Input: part model. Units: mm. Frame: model coordinates. A direction names the side the tool comes from. Round coordinates to 2 decimals unless told otherwise and drop trailing zeros. Loops run counter-clockwise (first coordinate to the right, second up) from the corner with the lowest first, then second, coordinate; pieces in that order, holes last. Notation, with made-up numbers: (-8, 41.5) -> (-2, 41.5) arc R27 cw to (-2, 63.5) -> close; hole circle Ø11 at (28, 45.5). An arc over 180 degrees is marked (long way). Answer in a Markdown table with one row per item. Add a question column.
Q1. Section B-B, the plane x = -37. Give the number of separate pieces and of enclosed holes in the cut face, and give its area (3 significant figures).
Q2. Reachability of faces 5 (the face through (-35, 1.5, -14)), 6 (the face through (-29.584, -2.107, 24.79)), 7 (the face through (-35, -6, 0)) from +Z, -Z, +X, -X, +Y, -Y: full face, straight path, thin tool, end or side. Return the list, or none.
Q3. Section D-D, the plane x = -28.25. Output: boundary loops of the cut face in (y, z), and give its area (3 significant figures).
Q4. Mould query, pull axis Z, two halves, no side actions, for faces 1 (the face through (-35, -1.494, -14)), 2 (the face through (-34.59, -0.03, -6.16)), 3 (the face through (-35, -6, 10)), 4 (the face through (-29.584, 2.107, -14.79)). Classes: pulls with the +Z half, pulls with the -Z half, needs draft (parallel to the pull), parting line crosses it, or undercut.
Q5. Pin query (flat end, axial travel): pin 1 (8 mm diameter, centred on x = -31.5, z = 28, fed in from +Y); pin 2 (5 mm diameter, centred on y = 2.5, z = -17, fed in from -X); pin 3 (8.5 mm diameter, centred on x = -37, z = -16.5, fed in from -Y). Return the tip coordinate at first contact, or that it passes through.
Q6. Section A-A, the plane z = 21.5. Output: boundary loops of the cut face in (x, y).
Q7. Ray query, L1, parallel to Z at x = -32, y = -0.25; L2, parallel to X at y = 0, z = 15.5; L3, parallel to Y at x = -34.75, z = -22. Return the intervals inside material, ascending. Write a range as from..to.
Q8. Section C-C, the plane z = -1.5. Output: boundary loops of the cut face in (x, y), and give its area (3 significant figures).
```python
from build123d import *

# Parameters (mm, degrees)
F0_R          = 8.5
F1_DEPTH      = 10
F2_R          = 5.5
F3_DEPTH      = 32
F4_R          = 5.5
F5_DEPTH      = 32
F6_SIZE       = 2
F7_SIZE       = 2
F8_R          = 3.0547772324
F9_DEPTH      = 8.501
F9_DEPTH_BACK = 8.501
F11_DEPTH     = 43.1654968794
F13_DEPTH     = 43.1654968794


with BuildPart() as f1:
    # F0 (on Top) → F1 (new body)
    with BuildSketch(Plane.XY):
        with Locations((-34.6644967794, 0)):
            Circle(F0_R)
    extrude(amount=F1_DEPTH)

    # F2 (on face) → F3 (join)
    with BuildSketch(Plane.XY.offset(10)):
        with Locations((-34.6644967794, 0)):
            Circle(F2_R)
    extrude(amount=F3_DEPTH)

    # F4 (on face) → F5 (join)
    with BuildSketch(Plane(origin=(0, 0, 0), x_dir=(1, 0, 0), z_dir=(0, 0, -1))):
        with Locations((-34.6644967794, 0)):
            Circle(F4_R)
    extrude(amount=F5_DEPTH)

    # F6
    f6_edges = [f1.edges().sort_by_distance(p)[0] for p in [
        (-40.164497, 0, 42),
    ]]
    chamfer(f6_edges, length=F6_SIZE)

    # F7
    f7_edges = [f1.edges().sort_by_distance(p)[0] for p in [
        (-40.164497, 0, -32),
    ]]
    chamfer(f7_edges, length=F7_SIZE)

    # F8 (on Front) → F9 (cut, two sides)
    with BuildSketch(Plane.XZ) as f9_sk:
        with Locations((-34.5804058015, 5.2290405147)):
            Circle(F8_R)
    extrude(amount=-F9_DEPTH, mode=Mode.SUBTRACT)
    extrude(f9_sk.sketch, amount=F9_DEPTH_BACK, mode=Mode.SUBTRACT)

    # F10 (on Right) → F11 (cut, through all)
    with BuildSketch(Plane.YZ):
        with BuildLine():
            Line((1.5, 20.7730699331), (1.5, 32.7730699331))
            ThreePointArc((1.5, 32.7730699331), (-0.0205803002, 34.2729287435), (-1.4994352683, 32.731913207))
            Line((-1.4994352683, 32.731913207), (-1.4994352683, 20.8142266592))
            Line((-1.4994352683, 20.8142266592), (-1.4994352683, 20.731913207))
            ThreePointArc((-1.4994352683, 20.731913207), (0.0205803002, 19.2732111226), (1.5, 20.7730699331))
        make_face()
        with BuildLine():
            Line((-1.4994352683, 20.731913207), (-1.4994352683, 20.8142266592))
            ThreePointArc((-1.4994352683, 20.8142266592), (-1.5, 20.7730699331), (-1.4994352683, 20.731913207))
        make_face()
    extrude(amount=-F11_DEPTH, mode=Mode.SUBTRACT)

    # F12 (on Right) → F13 (cut, through all)
    with BuildSketch(Plane.YZ):
        with BuildLine():
            Line((-1.4940902409, -19.792623133), (-1.4940902409, -19.5265828961))
            ThreePointArc((-1.4940902409, -19.5265828961), (-1.5, -19.6596030146), (-1.4940902409, -19.792623133))
        make_face()
        with BuildLine():
            Line((-1.4940902409, -7.792623133), (-1.4940902409, -19.5265828961))
            Line((-1.4940902409, -19.5265828961), (-1.4940902409, -19.792623133))
            ThreePointArc((-1.4940902409, -19.792623133), (0.0669880568, -21.1581064681), (1.4999997728, -19.6587774142))
            Line((1.4999997728, -19.6587774142), (1.5, -7.6596030146))
            ThreePointArc((1.5, -7.659603043), (-0.0665756517, -6.161081182), (-1.4940902409, -7.792623133))
        make_face()
    extrude(amount=-F13_DEPTH, mode=Mode.SUBTRACT)


solid = f1.part
```
Answer block:
| question | item | result |
|---|---|---|
| 1 | separate pieces | 2 |
| 1 | enclosed holes | 2 |
| 1 | area | 645 mm^2 |
| 2 | face 5 | +X, -X |
| 2 | face 6 | +Z |
| 2 | face 7 | -Z |
| 3 | outline | (-5.58, 0) -> (5.58, 0) -> (5.58, 10) -> (-5.58, 10) -> close |
| 3 | area | 112 mm^2 |
| 4 | face 1 | undercut |
| 4 | face 2 | undercut |
| 4 | face 3 | pulls with the +Z half |
| 4 | face 4 | needs draft |
| 5 | pin 1 | y = 5.5 |
| 5 | pin 2 | x = -39.96 |
| 5 | pin 3 | y = -5.5 |
| 6 | outline | (-39.96, -1.5) arc R5.5 ccw to (-29.37, -1.5) -> close; (-39.96, 1.5) -> (-29.37, 1.5) arc R5.5 ccw to start |
| 7 | L1 | -32..-21.14, -6.18..3.59, 6.86..19.29, 34.25..42 |
| 7 | L2 | -40.16..-29.16 |
| 7 | L3 | -5.5..5.5 |
| 8 | outline | circle Ø11 at (-34.66, 0) |
| 8 | area | 95.0 mm^2 |
